Autodesk Fusion 360 part; units mm, degrees
sketch "Schizzo1" plane through (0, 0, 0) normal (0, 0, 1) x (1, 0, 0)
  line L0 (0, 0) -> (90, 0)
  line L1 (90, 0) -> (90, 80)
  line L2 (90, 80) -> (0, 80)
  line L3 (0, 80) -> (0, 0)
  dimension "d1" = 90
  dimension "d2" = 80
extrude "Estrusione1" add sketch "Schizzo1" along normal blind 85
sketch "Schizzo2" plane through (0, 0, 0) normal (0, -1, 0) x (1, 0, 0)
  line L0 (0, 0) -> (90, 0)
  line L1 (90, 0) -> (90, 85)
  line L2 (90, 85) -> (0, 85)
  line L3 (0, 85) -> (0, 0)
  line L4 (90, 0) -> (90, 5)
  line L5 (90, 5) -> (0, 5)
  line L6 (0, 5) -> (0, 0)
  line L7 (0, 0) -> (90, 0)
  line L8 (0, 5) -> (37.3046, 85)
  line L9 (0, 5) -> (76.1109, 5) construction
  line L10 (37.3046, 85) -> (67.8203, 27.6084)
  line L11 (67.8203, 27.6084) -> (80.1815, 34.181)
  line L12 (80.1815, 34.181) -> (77.8342, 38.5957)
  line L13 (4.5315, 2.8869) -> (37.5979, 73.798)
  line L14 (37.5979, 73.798) -> (65.7529, 20.8463)
  line L15 (65.7529, 20.8463) -> (86.9436, 32.1136)
  line L16 (86.9436, 32.1136) -> (82.2489, 40.9431)
  line L17 (77.8342, 38.5957) -> (82.2489, 40.9431)
  line L18 (0, 5) -> (-2.3315, 0)
  line L19 (0, 0) -> (-2.3315, 0)
  dimension "d5" = 5
  dimension "d6" = 65
  dimension "d8" = 53
  dimension "d9" = 65
  dimension "d10" = 14
  dimension "d11" = 5
  dimension "d12" = 5
extrude "Estrusione2" cut sketch "Schizzo2" against normal blind 80 contours L2 L3 L8 | L1 L2 L5 L10 L11 L12 L13 L14 L15 L16 L17
fillet "Raccordo1" radius 15 1 edges at (5.5169, 40, 5)
fillet "Raccordo2" radius 15 1 edges at (37.5979, 40, 73.798)
fillet "Raccordo3" radius 2.6 6 edges at (80.1815, 40, 34.181) (77.8342, 40, 38.5957) (82.2489, 40, 40.9431) (67.8203, 40, 27.6084) (86.9436, 40, 32.1136) (65.7529, 40, 20.8463)
fillet "Raccordo4" radius 3 1 edges at (37.3046, 40, 85)
sketch "Schizzo3" plane through (0, 0, 0) normal (0, -1, 0) x (1, 0, 0)
  arc A0 (15.4676, 26.3393) -> (29.0622, 5) centre (29.0622, 20) ccw
  line L0 (15.4676, 26.3393) -> (24.8833, 46.5315)
  arc A1 (51.7222, 47.2343) -> (24.8833, 46.5315) centre (38.4779, 40.1922) ccw
  line L1 (51.7222, 47.2343) -> (64.5323, 23.142)
  arc A2 (64.5323, 23.142) -> (68.0485, 22.0669) centre (66.8279, 24.3626) ccw
  line L2 (68.0485, 22.0669) -> (84.648, 30.893)
  arc A3 (84.648, 30.893) -> (85.723, 34.4093) centre (83.4273, 33.1887) ccw
  line L3 (85.723, 34.4093) -> (84.0462, 37.5629)
  arc A4 (84.0462, 37.5629) -> (79.2079, 35.7992) centre (81.7505, 36.3423) ccw
  arc A5 (77.8859, 32.9604) -> (79.2079, 35.7992) centre (76.6652, 35.256) ccw
  line L4 (77.8859, 32.9604) -> (70.1159, 28.829)
  arc A6 (66.5996, 29.9041) -> (70.1159, 28.829) centre (68.8953, 31.1247) ccw
  line L5 (66.5996, 29.9041) -> (40.1295, 79.6872)
  arc A7 (40.1295, 79.6872) -> (34.7617, 79.5467) centre (37.4806, 78.2788) ccw
  line L6 (34.7617, 79.5467) -> (0, 5)
  line L7 (0, 5) -> (0, 0)
  line L8 (0, 0) -> (90, 0)
  line L9 (0, 5) -> (-2.8175, -1.0421)
  line L10 (0, 0) -> (-2.3315, 0)
  line L11 (90, 0) -> (90, 5)
  line L12 (90, 5) -> (29.0622, 5)
extrude "Estrusione3" add sketch "Schizzo3" against normal blind 80 contours L7 L9 L10
fillet "Raccordo6" radius 9 1 edges at (-2.3315, 40, 0)
sketch "Schizzo4" plane through (0, 0, 0) normal (0, -1, 0) x (1, 0, 0)
  arc A0 (3.6389, 12.8036) -> (11.7956, 0) centre (11.7956, 9) ccw
  line L0 (11.7956, 0) -> (90, 0)
  line L1 (90, 0) -> (90, 5)
  line L2 (90, 5) -> (29.0622, 5)
  arc A1 (15.4676, 26.3393) -> (29.0622, 5) centre (29.0622, 20) ccw
  line L3 (15.4676, 26.3393) -> (24.8833, 46.5315)
  arc A2 (51.7222, 47.2343) -> (24.8833, 46.5315) centre (38.4779, 40.1922) ccw
  line L4 (51.7222, 47.2343) -> (64.5323, 23.142)
  arc A3 (64.5323, 23.142) -> (68.0485, 22.0669) centre (66.8279, 24.3626) ccw
  line L5 (68.0485, 22.0669) -> (84.648, 30.893)
  arc A4 (84.648, 30.893) -> (85.723, 34.4093) centre (83.4273, 33.1887) ccw
  line L6 (85.723, 34.4093) -> (84.0462, 37.5629)
  arc A5 (84.0462, 37.5629) -> (79.2079, 35.7992) centre (81.7505, 36.3423) ccw
  arc A6 (77.8859, 32.9604) -> (79.2079, 35.7992) centre (76.6652, 35.256) ccw
  line L7 (77.8859, 32.9604) -> (70.1159, 28.829)
  arc A7 (66.5996, 29.9041) -> (70.1159, 28.829) centre (68.8953, 31.1247) ccw
  line L8 (66.5996, 29.9041) -> (40.1295, 79.6872)
  arc A8 (40.1295, 79.6872) -> (34.7617, 79.5467) centre (37.4806, 78.2788) ccw
  line L9 (34.7617, 79.5467) -> (3.6389, 12.8036)
  line L10 (100, -5) -> (83.9719, -5)
  line L11 (83.9719, -5) -> (83.9719, 13.2417)
  line L12 (83.9719, 13.2417) -> (100, 13.2417)
  line L13 (100, 13.2417) -> (100, -5)
extrude "Estrusione4" cut sketch "Schizzo4" against normal blind 80 contours L0 L1 L2 L11
fillet "Raccordo7" radius 2.2 2 edges at (83.9719, 40, 5) (83.9719, 40, 0)
sketch "Schizzo5" plane through (64.3166, 0, 34.1978) normal (0.8829, 0, 0.4695) x (0, 1, 0)
  line L0 (80, 51.52) -> (0, 51.52)
  line L1 (0, 51.52) -> (0, -4.8629)
  line L2 (0, -4.8629) -> (80, -4.8629)
  line L3 (80, -4.8629) -> (80, 51.52)
  circle A0 centre (40, 10) radius 20
  line L4 (20.0011, 9.7863) -> (20.3194, -19.9984)
  line L5 (60, 9.9667) -> (59.9501, -19.9992)
  line L6 (59.9501, -19.9992) -> (20.3194, -19.9984)
  line L7 (0, 0) -> (0, 10)
  line L8 (0, 10) -> (40, 10)
  dimension "d34" = 40
  dimension "d39" = 10
  dimension "d40" = 40
extrude "Estrusione5" cut sketch "Schizzo5" along normal blind 19 and the other way blind 15 contours L2 A0 L4 L5 L6 | L2 A0 L5 | L2 A0 | L2 A0 | L2 A0 L4
sketch "Schizzo6" plane through (0, 0, 0) normal (1, 0, 0) x (0, 1, 0)
  line L0 (80, 0) -> (80, 5)
  line L1 (80, 5) -> (40, 5)
  line L2 (40, 5) -> (40, 30)
  circle A0 centre (40, 30) radius 20
  line L3 (60, 30) -> (60, 5)
  line L4 (20, 30) -> (20, 5)
  line L5 (20, 5) -> (40, 5)
  dimension "d41" = 5
  dimension "d42" = 40
  dimension "d43" = 25
  dimension "d44" = 40
extrude "Estrusione6" cut sketch "Schizzo6" along normal blind 30
Design review of the part built by this model. Coordinates are the model's own, in mm. A direction names the side the tool comes from. Give positions to 0.01 mm unless a question says otherwise; leave off trailing zeros. Order: outer loops, then holes, each group sorted by start corner. A loop starts at its lowest first (then second) coordinate and runs counter-clockwise, first axis right, second up. Notation, with made-up numbers: (7, 51.25) - (40, 51.25) arc R20 cw to (40, 60.25) - close; hole circle Ø4 at (49, 20.25). An arc over 180 degrees is marked (long way). Write item = value, one per line. Start each with the question number.
Q1. Tool access review of faces 1 (the face through (76.2, 69.8, 26.4)), 2 (the face through (37.85, 40.56, 55.18)): name each direction out of +Z, -Z, +X, -X, +Y, -Y from which nothing blocks a thin tool from reaching the whole face with its end or side.
Q2. We need section A-A on x = 61. State the section outline as (y, z) points, plus the area to 3 significant figures.
Q3. Mouldability with a two-part tool opening along Z and no side actions: class faces 3 (the face through (84.895, 9.964, 35.966)), 4 (the face through (47, 39, 0)), 5 (the face through (85.922, 70.122, 32.456)), 6 (the face through (66.095, 10.261, 21.868)) as released by +Z, released by -Z, zero draft, split by the parting line, or undercut.
Q4. Clearance check with flat-ended pins moving along their axes: pin 1 Ø10 at (y, z) = (43, 42.5) entering from +X; pin 2 Ø4 at (y, z) = (12, 61) entering from +X; pin 3 Ø12 at (x, y) = (74.5, 19) entering from +Z. State where each tip first meets the part, or that it passes through.
Q5. To check wall thickness, follow L1, parallel to Y at x = 71, z = 25; L2, parallel to Z at x = 61.5, y = 44; L3, parallel to Z at x = 23, y = 33 (3 decimals). State the ranges of each line that lie inside material, in increasing order. Write a range as from..to.
Q6. We need section B-B on z = 65. State the section outline as (x, y) points, plus the area to 3 significant figures.
Working result:
q1.face_1 = +X, +Y, -Y
q1.face_2 = +Y, -Y
q2.outline = (0, 0) - (80, 0) - (80, 5) - (0, 5) - close; (0, 29.79) - (20.13, 29.79) - (20.03, 40.44) - (0, 40.44) - close; (59.98, 29.79) - (80, 29.79) - (80, 40.44) - (60, 40.44) - close
q2.area = 827 mm²
q3.face_3 = released by +Z
q3.face_4 = released by -Z
q3.face_5 = split by the parting line
q3.face_6 = undercut
q4.pin_1 = through
q4.pin_2 = 51.13
q4.pin_3 = 38.63
q5.L1 = 0..20.23, 59.96..80
q5.L2 = 0..5
q5.L3 = 0..5, 48.735..54.324
q6.outline = (27.98, 0) - (47.94, 0) - (47.94, 80) - (27.98, 80) - close
q6.area = 1,600 mm²
